Work out the finished part from the listing and answer in its coordinate system (mm). A direction names the side the tool comes from. Round coordinates to 2 decimals unless told otherwise and drop trailing zeros. Write each loop counter-clockwise with the first axis right and the second up, starting at its lowest first coordinate (ties: lowest second). Pieces come first, ordered by that corner, then holes. Notation, with made-up numbers: (42.25, 25) - (76.25, 25) arc R24 ccw to (76.25, 54) - close; hole circle Ø2 at (28.5, 63.5). An arc over 180 degrees is marked (long way). Answer as a JSON object with one key per item and string values.
```python
from build123d import *

# Parameters (mm, degrees)
F0_W     = 200
F0_H     = 150
F1_DEPTH = 100
F2_T     = -2.5
F3_R     = 5
F5_R     = 30
F6_DEPTH = 25
F7_T     = -2.5


with BuildPart() as f1:
    # F0 (on Top) → F1 (new body)
    with BuildSketch(Plane.XY):
        Rectangle(F0_W, F0_H)
    extrude(amount=F1_DEPTH)

    # F2
    f2_openings = [f1.faces().sort_by_distance(p)[0] for p in [
        (0, 0, 100),
    ]]
    offset(amount=F2_T, openings=f2_openings)

    # F3
    f3_edges = [f1.edges().sort_by_distance(p)[0] for p in [
        (-100, -75, 50),
        (-100, 75, 50),
        (100, 75, 50),
        (100, -75, 50),
    ]]
    fillet(f3_edges, radius=F3_R)


with BuildPart() as f6:
    # F5 (on Top) → F6 (new body)
    with BuildSketch(Plane.XY):
        Circle(F5_R)
    extrude(amount=F6_DEPTH)

    # F7
    f7_openings = [f6.faces().sort_by_distance(p)[0] for p in [
        (0, 0, 25),
    ]]
    offset(amount=F7_T, openings=f7_openings)


solid = f6.part
```
Item 1: Determine the mould class of faces 3 (the flat face through (13.2, -24.3, 25)), 4 (the cylindrical face through (-29.97, 1.32, 12.32)), 5 (the flat face through (0, 0, 2.5)) for opening direction X: pulls with the +X half, pulls with the -X half, needs draft (parallel to the pull), parting line crosses it, or undercut.
Results found:
{"face 3": "needs draft", "face 4": "parting line crosses it", "face 5": "undercut"}
Item 2: A cutting plane is placed at C-C (x = 3.5). Write down the section's boundary in (y, z).
Results found:
{"outline": "(-29.8, 0) - (29.8, 0) - (29.8, 25) - (27.28, 25) - (27.28, 2.5) - (-27.28, 2.5) - (-27.28, 25) - (-29.8, 25) - close"}
Item 3: A cutting plane is placed at B-B (y = 4). Write down the section's boundary in (x, z).
Results found:
{"outline": "(-29.73, 0) - (29.73, 0) - (29.73, 25) - (27.21, 25) - (27.21, 2.5) - (-27.21, 2.5) - (-27.21, 25) - (-29.73, 25) - close"}
Item 4: A cutting plane is placed at A-A (z = 3.75). Write down the section's boundary in (x, y), and give its area (3 significant figures).
Results found:
{"outline": "circle Ø60 at (0, 0); hole circle Ø55 at (0, 0)", "area": "452 mm²"}
Item 5: Consider line 1 along Y through (x, z) = (0, 12.5); line 2 along Z through (x, y) = (21.5, -9.5); line 3 along Y through (x, z) = (-6, 23). Determine where each line is inside the solid, lowest interval first.
Results found:
{"line 1": "-30 to -27.5, 27.5 to 30", "line 2": "0 to 2.5", "line 3": "-29.39 to -26.84, 26.84 to 29.39"}
Item 6: Each of these flat-tipped pins is pushed along its axis until it touches: P1, Ø12, axis at y = -18, z = 11.5, coming from the +X side; P2, Ø5, axis at y = -10, z = 11.5, coming from the -X side; P3, Ø2, axis at x = 20, z = 10, coming from the -Y side. Where does it stop, or does it pass through?
Results found:
{"P1": "x = 27.5", "P2": "x = -29.05", "P3": "y = -23.22"}
Item 7: For faces 1 (the cylindrical face through (-5.961, -26.846, 13.592)), 2 (the flat face through (0, 0, 0)), determine the directions among +Z, -Z, +X, -X, +Y, -Y from which every point of the face is accessible in a straight line to the end or side of a thin tool.
Results found:
{"face 1": "+Z", "face 2": "-Z, +X, -X, +Y, -Y"}
